Input: part model. Units: mm. Frame: model coordinates. A direction names the side the tool comes from. Round coordinates to 2 decimals unless told otherwise and drop trailing zeros. Order: outer loops, then holes, each group sorted by start corner. A loop starts at its lowest first (then second) coordinate and runs counter-clockwise, first axis right, second up. Notation, with made-up numbers: (13.25, 40.5) -> (47.25, 40.5) arc R23 ccw to (47.25, 55.5) -> close; hole circle Ø4 at (29, 32.25). An arc over 180 degrees is marked (long way). Use a Markdown table: item, result.
from build123d import *

# Parameters (mm, degrees)
SKETCH4_W                       = 48
SKETCH4_H                       = 70
SKETCH4_R                       = 22
BOSS_EXTRUDE2_DEPTH             = 10
SKETCH5_W                       = 5
SKETCH5_H                       = 55
CUT_EXTRUDE1_DEPTH              = 61.241181927
TAP_DRILL_FOR_M4X0_7_TAP1_D     = 3.3
TAP_DRILL_FOR_M4X0_7_TAP1_DEPTH = 10
TAP_DRILL_FOR_M4X0_7_TAP1_TIP   = 0.991420021


with BuildPart() as part:
    # Sketch4 → Boss-Extrude2 (new body)
    with BuildSketch(Plane(origin=(0, 0, 0), x_dir=(0, 0, -1), z_dir=(1, 0, 0))):
        Rectangle(SKETCH4_W, SKETCH4_H)
        with Locations((0, 11)):
            Circle(SKETCH4_R, mode=Mode.SUBTRACT)
    extrude(amount=BOSS_EXTRUDE2_DEPTH)

    # Sketch5 → Cut-Extrude1 (cut, through all)
    with BuildSketch(Plane(origin=(0, 0, -24), x_dir=(-1, 0, 0), z_dir=(0, 0, -1))):
        with Locations((-2.5, 7.5)):
            Rectangle(SKETCH5_W, SKETCH5_H)
    extrude(amount=-CUT_EXTRUDE1_DEPTH, mode=Mode.SUBTRACT)

    # Tap Drill for M4x0.7 Tap1
    with Locations(Plane(origin=(0, -35, 0), x_dir=(-1, 0, 0), z_dir=(0, -1, 0))):
        with Locations((-5, 19), (-5, -19)):
            Hole(TAP_DRILL_FOR_M4X0_7_TAP1_D / 2, depth=TAP_DRILL_FOR_M4X0_7_TAP1_DEPTH)
            with Locations((0, 0, -(TAP_DRILL_FOR_M4X0_7_TAP1_DEPTH + TAP_DRILL_FOR_M4X0_7_TAP1_TIP / 2))):  # 118° drill point
                Cone(0, TAP_DRILL_FOR_M4X0_7_TAP1_D / 2, TAP_DRILL_FOR_M4X0_7_TAP1_TIP, mode=Mode.SUBTRACT)


solid = part.part
1) Ray query, probe 1 along Z at (x, y) = (5, -32.5); probe 2 along X at (y, z) = (-30.5, 19); probe 3 along Y at (x, z) = (7.6, 0). Return the intervals inside material, ascending.
Answer key:
| item | result |
|---|---|
| probe 1 | z = -24 to -20.65, -17.35 to 17.35, 20.65 to 24 |
| probe 2 | x = 0 to 3.35, 6.65 to 10 |
| probe 3 | y = -35 to -11, 33 to 35 |
2) Cut plane C-C on y = -29. Return loops of the section in (x, z), and give its area (3 significant figures).
Answer key:
| item | result |
|---|---|
| outline | (0, -24) -> (10, -24) -> (10, 24) -> (0, 24) -> close; hole circle Ø3.3 at (5, -19); hole circle Ø3.3 at (5, 19) |
| area | 463 mm^2 |
3) Cut plane A-A on z = 0. Return loops of the section in (x, y), and give its area (3 significant figures).
Answer key:
| item | result |
|---|---|
| outline | (0, -35) -> (10, -35) -> (10, -11) -> (5, -11) -> (5, -20) -> (0, -20) -> close; (5, 33) -> (10, 33) -> (10, 35) -> (5, 35) -> close |
| area | 205 mm^2 |
4) Draft query along X for faces 4 (the face through (5, -11.2, -0.3)), 5 (the face through (5.04, -24.18, -19.28)), 6 (the face through (7, -8, -24)). Return one class per face: released by +X, released by -X, zero draft, split by the parting line, or undercut.
Answer key:
| item | result |
|---|---|
| face 4 | released by -X |
| face 5 | undercut |
| face 6 | zero draft |
5) Contact query for flat-ended pins moving along their axis: P1, Ø1.5, axis at x = 3.5, y = -5, coming from the +Z side; P2, Ø1.5, axis at x = 3, z = -4.5, coming from the +Y side; P3, Ø24, axis at y = 18.5, z = 7.5, coming from the -X side. Output: stop coordinate, or through.
Answer key:
| item | result |
|---|---|
| P1 | passes through |
| P2 | stops at y = -20 |
| P3 | stops at x = 5 |
6) Cut plane B-B on y = 11. Return loops of the section in (x, z).
Answer key:
| item | result |
|---|---|
| outline | (5, -24) -> (10, -24) -> (10, -22) -> (5, -22) -> close; (5, 22) -> (10, 22) -> (10, 24) -> (5, 24) -> close |
7) Cut plane D-D on x = 2.5. Return loops of the section in (y, z), and give its area (3 significant figures).
Answer key:
| item | result |
|---|---|
| outline | (-35, -24) -> (-20, -24) -> (-20, 24) -> (-35, 24) -> close |
| area | 720 mm^2 |
8) Set-up query: faces 1 (the face through (7.465, -10.477, 4.769)), 2 (the face through (3, -20, 0)), 3 (the face through (3.784, -29.93, 17.885)). Return all of +Z, -Z, +X, -X, +Y, -Y with unobstructed straight access to the full face (end or side cutting, diameter ignored); none if empty.
Answer key:
| item | result |
|---|---|
| face 1 | +X, -X |
| face 2 | +Z, -Z, -X, +Y |
| face 3 | -Y |
